from build123d import *

# Parameters (mm, degrees)
SKETCH1_W                    = 19.05
SKETCH1_H                    = 7.9248
SKETCH3_W                    = 12.7
SKETCH3_H                    = 7.9248
BOSS_EXTRUDE1_DEPTH          = 19.05
F_56_0_0465_DIAMETER_HOLE1_D = 1.1811


with BuildPart() as part:
    # Sweep1: sweep along a path in Sketch2
    with BuildLine(Plane(origin=(0, 0, 0), x_dir=(0, 0, -1), z_dir=(1, 0, 0))) as sweep1_path:
        ThreePointArc((0, 0), (-152.4, 152.4), (0, 304.8))
        Line((0, 304.8), (127, 304.8))
        ThreePointArc((127, 304.8), (198.842048969, 334.557951031), (228.6, 406.4))
    # Sketch1 → Sweep1 (sweep)
    with BuildSketch(Plane.XY):
        Rectangle(SKETCH1_W, SKETCH1_H)
    sweep(path=sweep1_path.line)

    # Sketch3 → Boss-Extrude1 (add)
    with BuildSketch(Plane(origin=(9.525, 0, 0), x_dir=(0, 0, -1), z_dir=(1, 0, 0))):
        with Locations((6.35, 0)):
            Rectangle(SKETCH3_W, SKETCH3_H)
    extrude(amount=-BOSS_EXTRUDE1_DEPTH)

    # #56 (0.0465) Diameter Hole1 (through all)
    with Locations(Plane(origin=(9.525, 0, 0), x_dir=(0, 0, -1), z_dir=(1, 0, 0))):
        with Locations((127, 304.8)):
            Hole(F_56_0_0465_DIAMETER_HOLE1_D / 2)


solid = part.part
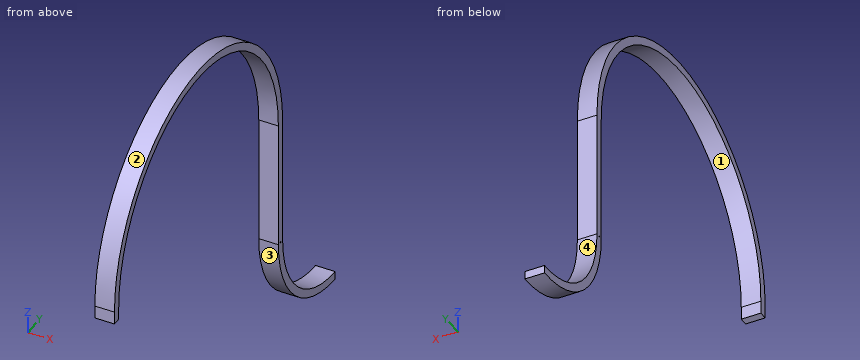
Could you check a few things on this model? Use its own coordinates, in mm. Face numbers are marked on the shaded views. Give positions to 0.01 mm unless a question says otherwise; leave off trailing zeros. Order: outer loops, then holes, each group sorted by start corner. A loop starts at its lowest first (then second) coordinate and runs counter-clockwise, first axis right, second up. Notation, with made-up numbers: (13.25, 43.5) - (42.25, 43.5) arc R34 cw to (42.25, 81.5) - close; hole circle Ø10 at (71, 73). An arc over 180 degrees is marked (long way). One line per item, written item: value. Start each with the question number.
1. Imagine slicing it at A-A on x = -5.5. List the corners of the cut face in (y, z) for me, plus the area to 3 significant figures.
2. Thinking about a two-plate mould opening in Y: for the marked faces 1, 2, 3 and 4, which applies, +Y half, -Y half, draft (parallel to the pull), parting line (faces both ways), or undercut?
3. Imagine slicing it at B-B on z = 46. List the corners of the cut face in (x, y) for me (3 decimals).
4. If I drill on probe 1 along Y at (x, z) = (-4.75, -127); probe 2 along Y at (x, z) = (-8, -10); probe 3 along Y at (x, z) = (-8.5, -129.5), over which ranges is the centre line in solid material (lowest first)?
5. For P1, Ø1.5, axis at x = 5.5, y = 215, coming from the +Z side; P2, Ø6.5, axis at x = -3.5, y = 1.5, coming from the -Z side; P3, Ø4, axis at x = 2.5, y = 334, coming from the +Z side; P4, Ø1.4, axis at y = 304.8, z = -127, coming from the -X side (3 decimals), each with a flat end and sliding along its axis, tell me the tip position at first contact or that it passes through.
6. Imagine slicing it at C-C on y = 152.4. List the corners of the cut face in (x, z) for me (3 decimals).
7. Imagine slicing it at D-D on z = -114.5. List the corners of the cut face in (x, y) for me (3 decimals).
Values:
1. outline: (-3.96, -12.7) - (3.96, -12.7) - (3.96, 0) arc R148.44 cw to (300.84, 0) - (300.84, -127) arc R105.56 ccw to (406.4, -232.56) - (406.4, -224.64) arc R97.64 cw to (308.76, -127) - (308.76, 0) arc R156.36 ccw to (-3.96, 0) - close; hole circle Ø1.18 at (304.8, -127)
1. area: 6,160 mm²
2. face 1: undercut
2. face 2: parting line
2. face 3: -Y half
2. face 4: +Y half
3. outline: (-9.525, 2.957) - (9.525, 2.957) - (9.525, 11.27) - (-9.525, 11.27) - close; (-9.525, 293.53) - (9.525, 293.53) - (9.525, 301.843) - (-9.525, 301.843) - close
4. probe 1: 300.84 to 304.21, 305.39 to 308.76
4. probe 2: -3.96 to 3.96, 300.84 to 308.76
4. probe 3: 300.87 to 308.79
5. P1: z = 143.61
5. P2: z = -12.7
5. P3: z = -190.23
5. P4: x = -9.525
6. outline: (-9.525, 148.438) - (9.525, 148.438) - (9.525, 156.362) - (-9.525, 156.362) - close
7. outline: (-9.525, 300.838) - (9.525, 300.838) - (9.525, 308.762) - (-9.525, 308.762) - close
